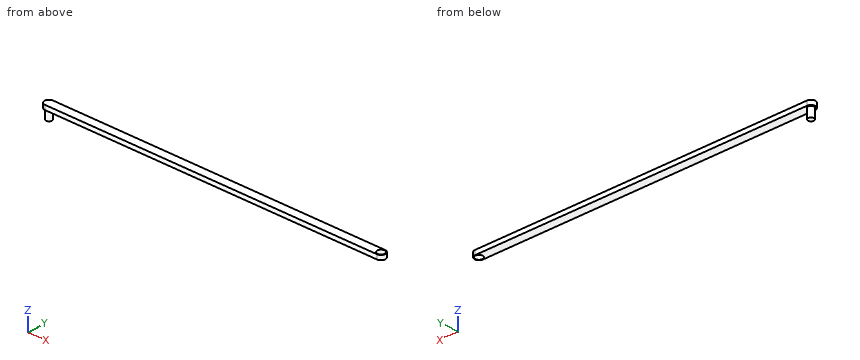
Autodesk Inventor part; units mm, degrees
ref_plane "YZ Plane" through (0, 0, 0) normal (1, 0, 0) x (0, 1, 0)
ref_plane "XZ Plane" through (0, 0, 0) normal (0, 1, 0) x (-1, 0, 0)
ref_plane "XY Plane" through (0, 0, 0) normal (0, 0, 1) x (1, 0, 0)
sketch "Boceto1" plane through (0, 0, 0) normal (0, 0, 1) x (1, 0, 0)
  arc A0 (0, 3.175) -> (0, -3.175) centre (0, 0) ccw
  arc A1 (240, -3.175) -> (240, 3.175) centre (240, 0) ccw
  line L0 (0, 3.175) -> (240, 3.175)
  line L1 (240, -3.175) -> (0, -3.175)
  dimension "d0" = 6.35
  dimension "d3" = 6.35
extrude "Extrusión1" add sketch "Boceto1" along normal blind 3.175
sketch "Boceto2" plane through (0, 0, 0) normal (0, 0, -1) x (-1, 0, 0)
  circle A0 centre (0, 0) radius 2.175
extrude "Extrusión2" add sketch "Boceto2" along normal blind 7
sketch "Boceto3" plane through (0, 0, 3.175) normal (0, 0, 1) x (1, 0, 0)
  arc A0 (240, -3.175) -> (240, 3.175) centre (240, 0) ccw
  circle A1 centre (240, 0) radius 3.175
  circle A2 centre (240, 0) radius 2.675
  point P0 (0, 0)
  dimension "d10" = 6.35
  dimension "d11" = 0.5
extrude "Extrusión3" cut sketch "Boceto3" against normal blind 5 contours A2
properties part number "eslabon_1" material "Aluminio 6061"
Geometry check sheet. Reference: the model listing, model coordinates, mm. Round coordinates to 2 decimals unless told otherwise and drop trailing zeros. Loops run counter-clockwise (first coordinate to the right, second up) from the corner with the lowest first, then second, coordinate; pieces in that order, holes last. Notation, with made-up numbers: M 41.25,37.5 L 89.25,37.5 A31 ccw 89.25,66.5 Z; hole C -38.5,35.25 d1. An arc over 180 degrees is marked long. Return JSON: item names as keys, results as strings. Group by question number.
(1) Section check C-C, the plane z = -1.75. Enter the section's corners in (x, y) (3 decimals), and give its area (3 significant figures).
(2) Scan lines: line 1 along Y through (x, z) = (240, 1.05) (3 decimals); line 2 along Z through (x, y) = (80, -0.25) (3 decimals); line 3 along X through (y, z) = (2, 2.5). Record each from-to range of solid material in increasing order. Write a range as [from, to].
(3) Go/stop test with flat-tipped pins: pin 1 (6 mm diameter, centred on x = 122, z = -5.5, fed in from -Y); pin 2 (2 mm diameter, centred on x = 33.5, y = 1.5, fed in from -Z). Record where each tip stops, or that it passes through.
(4) Section check B-B, the plane x = 107. Enter the section's corners in (y, z) (3 decimals).
(5) Section check A-A, the plane y = 1. Enter the section's corners in (x, z) (3 decimals).
Data:
{
 "1": {"outline": "C 0,0 d4.35", "area": "14.9 mm²"},
 "2": {"line 1": "[-3.175, -2.675], [2.675, 3.175]", "line 2": "[0, 3.175]", "line 3": "[-2.47, 238.22], [241.78, 242.47]"},
 "3": {"pin 1": "through", "pin 2": "z = 0"},
 "4": {"outline": "M -3.175,0 L 3.175,0 L 3.175,3.175 L -3.175,3.175 Z"},
 "5": {"outline": "M -3.013,0 L -1.931,0 L -1.931,-7 L 1.931,-7 L 1.931,0 L 237.519,0 L 237.519,3.175 L -3.013,3.175 Z; M 242.481,0 L 243.013,0 L 243.013,3.175 L 242.481,3.175 Z"}
}
